from build123d import *

# Parameters (mm, degrees)
F1_DEPTH = 750


with BuildPart() as f1:
    # F0 (on Top) → F1 (new body)
    with BuildSketch(Plane.XY):
        with BuildLine():
            Line((20, 5), (-20, 5))
            ThreePointArc((-20, 5), (-23.535534, 3.535534), (-25, 0))
            ThreePointArc((-25, 0), (-23.535534, -3.535534), (-20, -5))
            Line((-20, -5), (20, -5))
            ThreePointArc((20, -5), (23.535534, -3.535534), (25, 0))
            ThreePointArc((25, 0), (23.535534, 3.535534), (20, 5))
        make_face()
        with BuildLine():
            ThreePointArc((-23.9, 0), (-22.757716, 2.757716), (-20, 3.9))
            Line((-20, 3.9), (20, 3.9))
            ThreePointArc((20, 3.9), (22.757716, 2.757716), (23.9, 0))
            ThreePointArc((23.9, 0), (22.757716, -2.757716), (20, -3.9))
            Line((20, -3.9), (-20, -3.9))
            ThreePointArc((-20, -3.9), (-22.757716, -2.757716), (-23.9, 0))
        make_face(mode=Mode.SUBTRACT)
    extrude(amount=F1_DEPTH)


solid = f1.part
Could you check a few things on this model? Use its own coordinates, in mm. A direction names the side the tool comes from. Give positions to 0.01 mm unless a question says otherwise; leave off trailing zeros. Order: outer loops, then holes, each group sorted by start corner. A loop starts at its lowest first (then second) coordinate and runs counter-clockwise, first axis right, second up.
Item 1: I need wall thicknesses on line 1 (Y direction, x = 13, z = 394.5); line 2 (X direction, y = 0.75, z = 455); line 3 (X direction, y = -2.75, z = 207). Which ranges of each line are inside material? Lowest first, please.
Item 2: If we section it at A-A, the plane x = 1.5: Write out the boundary of the cut face in (y, z).
Item 3: I'm going to push flat-ended pins straight in: pin 1 (1 mm diameter, centred on y = 1.5, z = 284.5, fed in from +X); pin 2 (6 mm diameter, centred on y = -0.5, z = 101, fed in from -X); pin 3 (2 mm diameter, centred on y = 4, z = 88.5, fed in from +X). Where does each tip first touch, or does it pass through?
Item 4: If we mould it in two halves opening along X, with no side actions, what happens to faces 3 (the face through (0, 5, 370)), 4 (the face through (0, 3.9, 370))? For each: pulls with the +X half, pulls with the -X half, needs draft (parallel to the pull), parting line crosses it, or undercut.
Item 5: If we section it at B-B, the plane z = 469.5: Write out the boundary of the cut face in (x, y), plus the area to 3 significant figures.
Item 6: For faces 1 (the face through (0, -5, 370)), 2 (the face through (0, -3.9, 370)), which set-ups out of +Z, -Z, +X, -X, +Y, -Y let a thin tool reach every point of the face, with its end or its side?
Item 7: If we section it at C-C, the plane y = -1.75: Write out the boundary of the cut face in (x, z), plus the area to 3 significant figures.
Values:
1. line 1: y = -5 to -3.9, 3.9 to 5
1. line 2: x = -24.94 to -23.83, 23.83 to 24.94
1. line 3: x = -24.18 to -22.77, 22.77 to 24.18
2. outline: (-5, 0) - (-3.9, 0) - (-3.9, 750) - (-5, 750) - close; (3.9, 0) - (5, 0) - (5, 750) - (3.9, 750) - close
3. pin 1: stops at x = 24.9
3. pin 2: stops at x = -25
3. pin 3: stops at x = 24
4. face 3: needs draft
4. face 4: undercut
5. outline: (-20, -5) - (20, -5) arc R5 ccw to (20, 5) - (-20, 5) arc R5 ccw to start; hole (-23.9, 0) arc R3.9 ccw to (-20, -3.9) - (20, -3.9) arc R3.9 ccw to (23.9, 0) arc R3.9 ccw to (20, 3.9) - (-20, 3.9) arc R3.9 ccw to start
5. area: 119 mm2
6. face 1: +Z, -Z, +X, -X, -Y
6. face 2: +Z, -Z
7. outline: (-24.68, 0) - (-23.49, 0) - (-23.49, 750) - (-24.68, 750) - close; (23.49, 0) - (24.68, 0) - (24.68, 750) - (23.49, 750) - close
7. area: 1,800 mm2
